from build123d import *

# Parameters (mm, degrees)
BOSS_EXTRUDE1_DEPTH       = 12
M5X0_8_TAPPED_HOLE1_D     = 4.2
M5X0_8_TAPPED_HOLE1_DEPTH = 16
M5X0_8_TAPPED_HOLE1_TIP   = 1.2618073
M5X0_8_TAPPED_HOLE2_D     = 4.2
M5X0_8_TAPPED_HOLE2_DEPTH = 14
M5X0_8_TAPPED_HOLE2_TIP   = 1.2618073


with BuildPart() as part:
    # Sketch1 → Boss-Extrude1 (new body)
    with BuildSketch(Plane.XY):
        Polygon((15, 104.5), (35, 84.5), (35, 0), (5, 0), (0, 5), (0, 104.5), align=None)
    extrude(amount=BOSS_EXTRUDE1_DEPTH)

    # M5x0.8 Tapped Hole1
    with Locations(Plane.ZY):
        with Locations((6, 90), (6, 20)):
            Hole(M5X0_8_TAPPED_HOLE1_D / 2, depth=M5X0_8_TAPPED_HOLE1_DEPTH)
            with Locations((0, 0, -(M5X0_8_TAPPED_HOLE1_DEPTH + M5X0_8_TAPPED_HOLE1_TIP / 2))):  # 118° drill point
                Cone(0, M5X0_8_TAPPED_HOLE1_D / 2, M5X0_8_TAPPED_HOLE1_TIP, mode=Mode.SUBTRACT)

    # M5x0.8 Tapped Hole2
    with Locations(Plane.XZ):
        with Locations((25, 6)):
            Hole(M5X0_8_TAPPED_HOLE2_D / 2, depth=M5X0_8_TAPPED_HOLE2_DEPTH)
            with Locations((0, 0, -(M5X0_8_TAPPED_HOLE2_DEPTH + M5X0_8_TAPPED_HOLE2_TIP / 2))):  # 118° drill point
                Cone(0, M5X0_8_TAPPED_HOLE2_D / 2, M5X0_8_TAPPED_HOLE2_TIP, mode=Mode.SUBTRACT)


solid = part.part
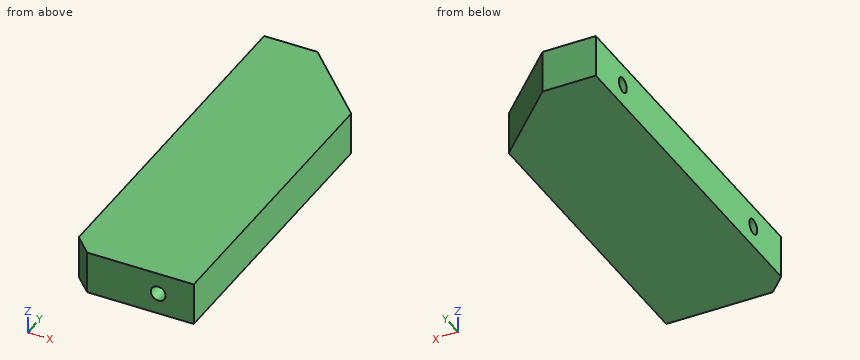
The model under review builds one solid part; all positions refer to its coordinate system, in mm. Give positions to 0.01 mm unless a question says otherwise; leave off trailing zeros. Loops run counter-clockwise (first coordinate to the right, second up) from the corner with the lowest first, then second, coordinate; pieces in that order, holes last. Notation, with made-up numbers: (-8, 24) -> (15, 24) arc R7 cw to (15, 32) -> close; hole circle Ø4 at (74, 5). An arc over 180 degrees is marked (long way). Answer as a JSON object with one key per item and string values. Group by question number.
Q1. Take a section at C-C (y = 86). Write out the cut boundary in (x, z).
Q2. Take a section at A-A (x = 4). Write out the cut boundary in (y, z), plus the area to 3 significant figures.
Q3. Wall thickness on line 1 along Y through (x, z) = (7, 6); line 2 along X through (y, z) = (9.25, 6); line 3 along Y through (x, z) = (8, 7.25): over which ranges is each line inside the solid? List them lowest first.
Q4. Insertion check: pin 1 (6 mm diameter, centred on x = 25, z = 4, fed in from +Y); pin 2 (2.5 mm diameter, centred on y = 90, z = 6, fed in from +X); pin 3 (4 mm diameter, centred on y = 20, z = 6, fed in from -X). Each pin has a flat end and moves straight along its axis. Give the tip position at first contact, or say it passes through.
Q5. Take a section at B-B (x = 19). Write out the cut boundary in (y, z), plus the area to 3 significant figures.
Answer below:
{
 "1": {"outline": "(0, 0) -> (33.5, 0) -> (33.5, 12) -> (0, 12) -> close"},
 "2": {"outline": "(1, 0) -> (104.5, 0) -> (104.5, 12) -> (1, 12) -> close; hole circle Ø4.2 at (20, 6); hole circle Ø4.2 at (90, 6)", "area": "1,210 mm2"},
 "3": {"line 1": "y = 0 to 17.9, 22.1 to 87.9, 92.1 to 104.5", "line 2": "x = 0 to 22.9, 27.1 to 35", "line 3": "y = 0 to 18.31, 21.69 to 88.31, 91.69 to 104.5"},
 "4": {"pin 1": "stops at y = 97.5", "pin 2": "stops at x = 30.75", "pin 3": "stops at x = 16.06"},
 "5": {"outline": "(0, 0) -> (100.5, 0) -> (100.5, 12) -> (0, 12) -> close", "area": "1,210 mm2"}
}
